```python
from build123d import *

# Parameters (mm, degrees)
CROQUIS1_R              = 11
CROQUIS1_R_2            = 4
SALIENTE_EXTRUIR1_DEPTH = 6.95
CHAFL_N1_SIZE           = 0.25
CHAFL_N2_SIZE           = 0.25
CHAFL_N2_SIZE2          = 0.144337567


with BuildPart() as part:
    # Croquis1 → Saliente-Extruir1 (new body)
    with BuildSketch(Plane(origin=(0, 0, 0), x_dir=(1, 0, 0), z_dir=(0, 1, 0))):
        with Locations(Location((0, 0, 0), (0, 0, 270))):
            Circle(CROQUIS1_R)
        with Locations(Location((0, 0, 0), (0, 0, 270))):
            Circle(CROQUIS1_R_2, mode=Mode.SUBTRACT)
    extrude(amount=SALIENTE_EXTRUIR1_DEPTH)

    # Croquis2 → Cortar-Revolución1 (revolve, cut)
    with BuildSketch(Plane.XY, mode=Mode.PRIVATE) as cortar_revoluci_n1_sk:
        Polygon((-9.75, 6.95), (-9.75, 5.95), (-8.85, 6.85), (-6.15, 6.85), (-6.15, 6.45), (-5.65, 6.95), align=None)
        Polygon((-8.85, 0.1), (-6.15, 0.1), (-6.15, 0.5), (-5.65, 0), (-9.75, 0), (-9.75, 1), align=None)
    revolve(cortar_revoluci_n1_sk.sketch.rotate(Axis((0, 0, 0), (0, 1, 0)), 270), axis=Axis((0, 0, 0), (0, 1, 0)), mode=Mode.SUBTRACT)

    # Chaflán1
    chafl_n1_edges = [part.edges().sort_by_distance(p)[0] for p in [
        (0, 0, -4),
        (0, 6.95, -4),
    ]]
    chamfer(chafl_n1_edges, length=CHAFL_N1_SIZE)

    # Chaflán2
    chafl_n2_edges = [part.edges().sort_by_distance(p)[0] for p in [
        (0, 0, -11),
        (0, 6.95, -11),
    ]]
    chafl_n2_side = [part.faces().sort_by_distance(p)[0] for p in [
        (0, 3.475, -11),
    ]]
    chamfer(chafl_n2_edges, length=CHAFL_N2_SIZE, length2=CHAFL_N2_SIZE2, reference=chafl_n2_side[0])


solid = part.part
```
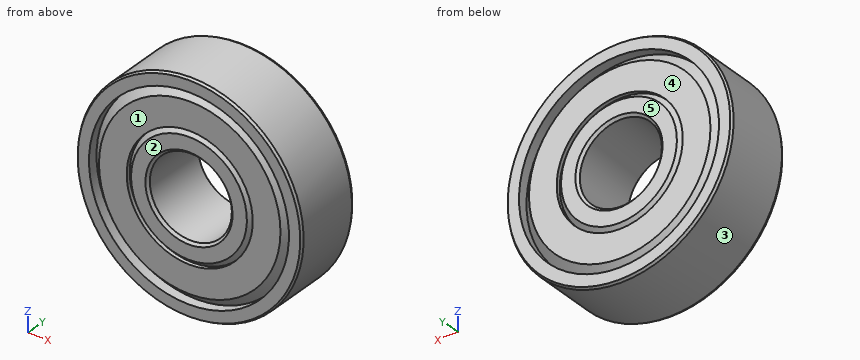
The listing builds one solid part. Answer for the finished solid, in the listing's coordinates (mm). Face numbers are marked on the shaded views. A direction names the side the tool comes from. Give positions to 0.01 mm unless a question says otherwise; leave off trailing zeros. Order: outer loops, then holes, each group sorted by start corner. A loop starts at its lowest first (then second) coordinate and runs counter-clockwise, first axis right, second up. Notation, with made-up numbers: (62.5, 28) - (70.5, 28) arc R23 ccw to (70.5, 46) - close; hole circle Ø11 at (65, 5.25). An arc over 180 degrees is marked (long way). Answer in a Markdown table with one row per item. Add a question column.
Q1. The part is cut by section A-A (y = 3.25). Determine the outline of the cut face in (x, z).
Q2. Given P1, Ø1, axis at y = 1, z = -1.5, coming from the -X side; P2, Ø4, axis at x = -4.5, y = 1.5, coming from the +Z side; P3, Ø1, axis at x = -2.5, z = 6, coming from the +Y side, each flat-ended and moving along its own axis, determine where each tip first touches the part or whether it passes through.
Q3. Which of the six approach directions +Z, -Z, +X, -X, +Y, -Y give full straight-line access (tool end or side, diameter ignored) to the marked faces 4 and 5?
Q4. For a pull along Z with two mould halves and no side action, classify the marked faces 1, 2 and 3 as released by +Z, released by -Z, zero draft, split by the parting line, or undercut.
Q5. Find the intervals of material crossed by line 1 along X through (y, z) = (0.5, -6.5); line 2 along X through (y, z) = (5.25, 2.5); line 3 along X through (y, z) = (5.75, 2.25), in increasing order. Write a range as [from, to].
Determined:
| question | item | result |
|---|---|---|
| 1 | outline | circle Ø22 at (0, 0); hole circle Ø8 at (0, 0) |
| 2 | P1 | stops at x = -10.95 |
| 2 | P2 | stops at z = 10.71 |
| 2 | P3 | stops at y = 6.85 |
| 3 | face 4 | +Y |
| 3 | face 5 | +Z, -Z, +X, -X, +Y |
| 4 | face 1 | undercut |
| 4 | face 2 | zero draft |
| 4 | face 3 | split by the parting line |
| 5 | line 1 | x = [-8.87, -7.27], [-6.58, 6.58], [7.27, 8.87] |
| 5 | line 2 | x = [-10.71, -3.12], [3.12, 10.71] |
| 5 | line 3 | x = [-10.77, -3.31], [3.31, 10.77] |
